```python
from build123d import *

# Parameters (mm, degrees)
SKETCH1_R           = 4
BOSS_EXTRUDE1_DEPTH = 75
SKETCH2_R           = 2.5
CUT_EXTRUDE1_DEPTH  = 1097
SKETCH3_W           = 40.4
SKETCH3_H           = 41.541480206
CUT_EXTRUDE2_DEPTH  = 5


with BuildPart() as part:
    # Sketch1 → Boss-Extrude1 (new body, symmetric)
    with BuildSketch(Plane(origin=(0, 0, 0), x_dir=(0, 0, -1), z_dir=(1, 0, 0))):
        Circle(SKETCH1_R)
    extrude(amount=BOSS_EXTRUDE1_DEPTH, both=True)

    # Sketch2 → Cut-Extrude1 (cut)
    with BuildSketch(Plane(origin=(-1373.627106081, 398.034078038, -1457.249478015), x_dir=(0, 0.520791654, 0.853683813), z_dir=(0, -0.853683813, 0.520791654))):
        with Locations((1036.737465208, -1406.127106081)):
            Circle(SKETCH2_R)
    extrude(amount=CUT_EXTRUDE1_DEPTH, mode=Mode.SUBTRACT)

    # Sketch3 → Cut-Extrude2 (cut, symmetric)
    with BuildSketch(Plane(origin=(0, 0, 0), x_dir=(1, 0, 0), z_dir=(0, 1, 0))):
        with Locations((75, 4)):
            Rectangle(SKETCH3_W, SKETCH3_H)
    extrude(amount=CUT_EXTRUDE2_DEPTH, both=True, mode=Mode.SUBTRACT)


solid = part.part
```
Work out the finished part from the listing and answer in its coordinate system (mm). A direction names the side the tool comes from. Give positions to 0.01 mm unless a question says otherwise; leave off trailing zeros. Write each loop counter-clockwise with the first axis right and the second up, starting at its lowest first coordinate (ties: lowest second). Pieces come first, ordered by that corner, then holes.
(1) The part is cut by section B-B on y = -2.5. Write down the section's boundary in (x, z), plus the area to 3 significant figures.
Final values:
outline: (-75, -3.12) - (54.8, -3.12) - (54.8, 3.12) - (-75, 3.12) - close
area: 811 mm2
(2) Straight lines are drawn through the part: line 1 (X direction, y = 1.5, z = -1.5); line 2 (Z direction, x = 3.5, y = 2.75); line 3 (Y direction, x = -46, z = 0.5). For each, find the intervals that lie inside material, in ascending order.
Final values:
line 1: x = -75 to 30.05, 34.95 to 54.8
line 2: z = -2.9 to 2.9
line 3: y = -3.97 to 3.97
(3) The part is cut by section A-A on x = -42. Write down the section's boundary in (y, z).
Final values:
outline: circle Ø8 at (0, 0)
(4) Which of the six approach directions +Z, -Z, +X, -X, +Y, -Y give full straight-line access (tool end or side, diameter ignored) to faces 1 (the flat face through (54.8, 0, 0)), 2 (the flat face through (32.46, 1.45, -0.92))?
Final values:
face 1: +Z, -Z, +X, +Y, -Y
face 2: none
(5) Flat-ended cylindrical pins translate along their axes: pin 1 Ø1.5 at (x, y) = (-8.5, -2) entering from +Z; pin 2 Ø1.5 at (x, z) = (-13, -1.5) entering from +Y. Find the tip coordinate at first contact, or state that the pin passes through.
Final values:
pin 1: stops at z = 3.8
pin 2: stops at y = 3.93
(6) The mould has two halves that part along Z. Classify faces 3 (the cylindrical face through (31.75, 3.48, 0.67)), 4 (the flat face through (-75, 0, 0)), 5 (the cylindrical face through (-9.191, -3.905, 0.867)): pulls with the +Z half, pulls with the -Z half, needs draft (parallel to the pull), parting line crosses it, or undercut.
Final values:
face 3: undercut
face 4: needs draft
face 5: parting line crosses it
